from build123d import *

# Parameters (mm, degrees)
SKETCH_1_W          = 35.7
SKETCH_1_H          = 29
EXTRUDE_1_DEPTH     = 6
SKETCH_2_R          = 1.55
CUT_EXTRUDE_1_DEPTH = 6
SKETCH_3_W          = 22.7
SKETCH_3_H          = 24
CUT_EXTRUDE_2_DEPTH = 10
FILLET_1_R          = 2


with BuildPart() as part:
    # 草图1 → 凸台-拉伸1 (new body)
    with BuildSketch(Plane.XY):
        Rectangle(SKETCH_1_W, SKETCH_1_H)
    extrude(amount=EXTRUDE_1_DEPTH)

    # 草图2 → 切除-拉伸1 (cut)
    with BuildSketch(Plane(origin=(0, 0, 0), x_dir=(-1, 0, 0), z_dir=(0, 0, -1))):
        with Locations((14.35, 0)):
            Circle(SKETCH_2_R)
        with Locations((-14.35, 10)):
            Circle(SKETCH_2_R)
        with Locations((-14.35, -10)):
            Circle(SKETCH_2_R)
    extrude(amount=-CUT_EXTRUDE_1_DEPTH, mode=Mode.SUBTRACT)

    # 草图3 → 切除-拉伸2 (cut)
    with BuildSketch(Plane(origin=(0, 0, 0), x_dir=(-1, 0, 0), z_dir=(0, 0, -1))):
        Rectangle(SKETCH_3_W, SKETCH_3_H)
    extrude(amount=-CUT_EXTRUDE_2_DEPTH, mode=Mode.SUBTRACT)

    # 圆角1
    fillet_1_edges = [part.edges().sort_by_distance(p)[0] for p in [
        (-11.35, 12, 3),
        (-11.35, -12, 3),
        (11.35, -12, 3),
        (11.35, 12, 3),
        (17.85, -14.5, 3),
        (-17.85, -14.5, 3),
        (-17.85, 14.5, 3),
        (17.85, 14.5, 3),
    ]]
    fillet(fillet_1_edges, radius=FILLET_1_R)


solid = part.part
Verification items for the finished model (mm, model axes). A direction names the side the tool comes from. Round coordinates to 2 decimals unless told otherwise and drop trailing zeros. Loops run counter-clockwise (first coordinate to the right, second up) from the corner with the lowest first, then second, coordinate; pieces in that order, holes last. Notation, with made-up numbers: (-9.5, 33.25) - (46.5, 33.25) arc R33 cw to (46.5, 62.25) - close; hole circle Ø7 at (-30, 36). An arc over 180 degrees is marked (long way). Write item = value, one per line.
Q1. Material ranges on L1, parallel to Y at x = 14.35, z = 4.6; L2, parallel to X at y = -2.75, z = 5.55; L3, parallel to Y at x = 2.5, z = 0.5, recorded low to high.
Here are the results:
L1 = -14.5 to -11.55, -8.45 to 8.45, 11.55 to 14.5
L2 = -17.85 to -11.35, 11.35 to 17.85
L3 = -14.5 to -12, 12 to 14.5
Q2. Tool access check on faces 1 (the cylindrical face through (10.78, -11.4, 3.04)), 2 (the flat face through (-12, 0, 6)). Record the directions out of +Z, -Z, +X, -X, +Y, -Y that give a thin tool (end or side, any length) a straight path to the whole face; none if there is none.
Here are the results:
face_1 = +Z, -Z
face_2 = +Z, +X, -X, +Y, -Y
Q3. Sectioned sample at D-D on x = 14.35. Record the boundary of the cut face in (y, z).
Here are the results:
outline = (-14.5, 0) - (-11.55, 0) - (-11.55, 6) - (-14.5, 6) - close; (-8.45, 0) - (8.45, 0) - (8.45, 6) - (-8.45, 6) - close; (11.55, 0) - (14.5, 0) - (14.5, 6) - (11.55, 6) - close
Q4. Sectioned sample at B-B on z = 2.9. Record the boundary of the cut face in (x, y).
Here are the results:
outline = (-17.85, -12.5) arc R2 ccw to (-15.85, -14.5) - (15.85, -14.5) arc R2 ccw to (17.85, -12.5) - (17.85, 12.5) arc R2 ccw to (15.85, 14.5) - (-15.85, 14.5) arc R2 ccw to (-17.85, 12.5) - close; hole circle Ø3.1 at (-14.35, 0); hole (-11.35, -10) arc R2 ccw to (-9.35, -12) - (9.35, -12) arc R2 ccw to (11.35, -10) - (11.35, 10) arc R2 ccw to (9.35, 12) - (-9.35, 12) arc R2 ccw to (-11.35, 10) - close; hole circle Ø3.1 at (14.35, -10); hole circle Ø3.1 at (14.35, 10)
Q5. Sectioned sample at A-A on x = -14.35. Record the boundary of the cut face in (y, z), plus the area to 3 significant figures.
Here are the results:
outline = (-14.5, 0) - (-1.55, 0) - (-1.55, 6) - (-14.5, 6) - close; (1.55, 0) - (14.5, 0) - (14.5, 6) - (1.55, 6) - close
area = 155 mm^2
Q6. Sectioned sample at C-C on y = 4. Record the boundary of the cut face in (x, z), plus the area to 3 significant figures.
Here are the results:
outline = (-17.85, 0) - (-11.35, 0) - (-11.35, 6) - (-17.85, 6) - close; (11.35, 0) - (17.85, 0) - (17.85, 6) - (11.35, 6) - close
area = 78.0 mm^2
Q7. Mould release check, pull along Y, two halves, no side actions. Record for faces 3 (the cylindrical face through (17.25, -13.93, 3.04)), 4 (the flat face through (17.85, 0, 3)), 5 (the flat face through (11.35, 0, 3)), 6 (the flat face through (0, 12, 3)): +Y half, -Y half, draft (parallel to the pull), parting line (faces both ways), or undercut.
Here are the results:
face_3 = -Y half
face_4 = draft
face_5 = undercut
face_6 = undercut
